For this review, take the finished solid that the model builds, in its own axes (mm). Give positions to 0.01 mm unless a question says otherwise; leave off trailing zeros. Loops run counter-clockwise (first coordinate to the right, second up) from the corner with the lowest first, then second, coordinate; pieces in that order, holes last. Notation, with made-up numbers: (87, -26.75) - (144, -26.75) arc R8 cw to (144, -20.75) - close; hole circle Ø4 at (64.5, 10). An arc over 180 degrees is marked (long way). Use CSV: the item, a comma, the result in double quotes. Start each with the question number.
1. Wall thickness on line 1 (Z direction, x = 6.5, y = 170.5); line 2 (X direction, y = 65, z = -7); line 3 (Z direction, x = 9, y = 82): over which ranges is each line inside the solid? List them lowest first.
2. For pin 1 (11.5 mm diameter, centred on y = 141.5, z = 15, fed in from +X); pin 2 (6 mm diameter, centred on x = -0.5, z = 5, fed in from +Y); pin 3 (8 mm diameter, centred on y = 125.5, z = -11.5, fed in from -X); pin 4 (12 mm diameter, centred on x = -8, y = 52.5, fed in from -Z), all flat-tipped, find the tip position at first contact; note any pin that passes through.
3. Take a section at B-B on z = 11.5. Give the boundary of the cut face in (x, y).
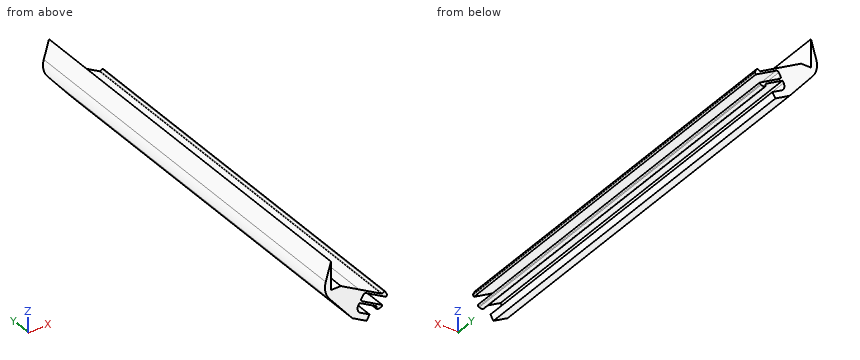
```python
from build123d import *

# Parameters (mm, degrees)
BOSS_EXTRUDE1_DEPTH   = 200
BOSS_EXTRUDE1_2_DEPTH = 200
FILLET1_R             = 0.5
FILLET2_R             = 0.5
BOSS_EXTRUDE3_DEPTH   = 200
FILLET3_R             = 10
FILLET4_R             = 1
FILLET5_R             = 3


with BuildPart() as part:
    # Sketch1 → Boss-Extrude1 (new body)
    with BuildSketch(Plane(origin=(0, 0, 0), x_dir=(1, 0, 0), z_dir=(0, 1, 0))):
        Polygon((13.927082127, 14.175350351), (16.351953258, 13.843299543), (16.851953258, 12.977274139), (3.059579159, 5.014243241), (2.594699496, 5.900545381), (13.927082127, 12.443299543), align=None)
    extrude(amount=BOSS_EXTRUDE1_DEPTH)

    # Fillet2
    fillet2_edges = [part.edges().sort_by_distance(p)[0] for p in [
        (13.927082127, 100, -14.175350351),
        (16.351953258, 100, -13.843299543),
        (13.927082127, 100, -12.443299543),
    ]]
    fillet(fillet2_edges, radius=FILLET2_R)



with BuildPart() as body_2:
    # Sketch1 → Boss-Extrude1 2 (new body)
    with BuildSketch(Plane(origin=(0, 0, 0), x_dir=(1, 0, 0), z_dir=(0, 1, 0))):
        Polygon((18.751953258, 9.686377605), (19.251953258, 8.820352201), (18.153877046, 6.454326797), (16.653877046, 7.320352201), (5.114206816, 0.657920487), (4.719127398, 1.584521817), align=None)
    extrude(amount=BOSS_EXTRUDE1_2_DEPTH)

    # Fillet1
    fillet1_edges = [body_2.edges().sort_by_distance(p)[0] for p in [
        (19.251953258, 100, -8.820352201),
        (18.153877046, 100, -6.454326797),
        (16.653877046, 100, -7.320352201),
    ]]
    fillet(fillet1_edges, radius=FILLET1_R)


with BuildPart() as part_1:
    add(part.part)

    add(body_2.part)  # Boss-Extrude3 merges body 2
    # Sketch2 → Boss-Extrude3 (add)
    with BuildSketch(Plane(origin=(0, 0, 0), x_dir=(1, 0, 0), z_dir=(0, 1, 0))):
        Polygon((8.182648293, 2.429486), (3.232648293, 11.003137498), (10.393111947, 15.137233116), (8.893111947, 17.735309327), (1.732648293, 13.601213709), (-13.163737181, -4.647533202), (-9.075108531, -18.787281313), (-9.075108531, -4.647533202), (-4.075108531, -4.647533202), align=None)
    extrude(amount=BOSS_EXTRUDE3_DEPTH)

    # Fillet3
    fillet3_edges = [part_1.edges().sort_by_distance(p)[0] for p in [
        (-13.163737181, 100, 4.647533202),
    ]]
    fillet(fillet3_edges, radius=FILLET3_R)

    # Fillet4
    fillet4_edges = [part_1.edges().sort_by_distance(p)[0] for p in [
        (5.782648293, 100, -6.586407938),
        (7.682648293, 100, -3.295511404),
    ]]
    fillet(fillet4_edges, radius=FILLET4_R)

    # Fillet5
    fillet5_edges = [part_1.edges().sort_by_distance(p)[0] for p in [
        (3.232648293, 100, -11.003137498),
    ]]
    fillet(fillet5_edges, radius=FILLET5_R)


solid = part_1.part
```
Check result:
1,line 1,"z = -16.35 to -12.89, -8.16 to -6.98, -5.34 to -1.46"
1,line 2,"x = -3.66 to 6.52, 14.1 to 16.1, 17.21 to 18.41"
1,line 3,"z = -17.55 to -14.33, -9.6 to -8.44, -4.06 to -2.9"
2,pin 1,"stops at x = -9.08"
2,pin 2,"stops at y = 200"
2,pin 3,"stops at x = -3.25"
2,pin 4,"stops at z = -9.03"
3,outline,"(-11.18, 0) - (-9.08, 0) - (-9.08, 200) - (-11.18, 200) - close"
